CAD build for the part. Positions are in the model's coordinates, mm. A direction names the side the tool comes from. Round coordinates to 2 decimals unless told otherwise and drop trailing zeros. Loops run counter-clockwise (first coordinate to the right, second up) from the corner with the lowest first, then second, coordinate; pieces in that order, holes last.
from build123d import *

# Parameters (mm, degrees)
SKETCH1_R      = 53.975
SKETCH1_R_2    = 50.8
EXTRUDE1_DEPTH = 304.8
SKETCH2_W      = 76.2
SKETCH2_H      = 203.2
EXTRUDE2_DEPTH = 315.212732476
FILLET1_R      = 6.35


with BuildPart() as part:
    # Sketch1 → Extrude1 (new body)
    with BuildSketch(Plane.XY):
        with Locations(Location((0, 0, 0), (0, 0, 180))):
            Circle(SKETCH1_R)
        with Locations(Location((0, 0, 0), (0, 0, 180))):
            Circle(SKETCH1_R_2, mode=Mode.SUBTRACT)
    extrude(amount=EXTRUDE1_DEPTH)

    # Sketch2 → Extrude2 (cut, through all)
    with BuildSketch(Plane(origin=(0, 0, 0), x_dir=(1, 0, 0), z_dir=(0, 1, 0))):
        with Locations((0, -152.4)):
            Rectangle(SKETCH2_W, SKETCH2_H)
    extrude(amount=-EXTRUDE2_DEPTH, mode=Mode.SUBTRACT)

    # Fillet1
    # the kernel refuses this fillet: 6.35 mm, written as the material it adds along each edge
    with BuildSketch(Plane(origin=(-38.1, -17.726041651, 254), x_dir=(0, 0, -1), z_dir=(0, -1, 0))) as fillet1_piece_1_section:
        with BuildLine():
            CenterArc((FILLET1_R, FILLET1_R), FILLET1_R, 180, 90)
            Line((0, FILLET1_R), (0, 0))
            Line((0, 0), (FILLET1_R, 0))
        make_face()
    fillet1_piece_1 = extrude(amount=36.381021137, mode=Mode.PRIVATE)
    fillet1_piece_1 = fillet1_piece_1 & Plane(origin=(0, 0, 252.560306593), x_dir=(-1, 0, 0), z_dir=(0, 0, -1)) * Cylinder(53.975, 99, mode=Mode.PRIVATE)
    fillet1_piece_1 = fillet1_piece_1 - Plane(origin=(0, 0, 252.560306593), x_dir=(-1, 0, 0), z_dir=(0, 0, -1)) * Cylinder(50.8, 99, mode=Mode.PRIVATE)
    add(fillet1_piece_1)
    with BuildSketch(Plane(origin=(-38.1, -17.726041651, 50.8), x_dir=(1, 0, 0), z_dir=(0, -1, 0))) as fillet1_piece_2_section:
        with BuildLine():
            CenterArc((FILLET1_R, FILLET1_R), FILLET1_R, 180, 90)
            Line((0, FILLET1_R), (0, 0))
            Line((0, 0), (FILLET1_R, 0))
        make_face()
    fillet1_piece_2 = extrude(amount=36.381021137, mode=Mode.PRIVATE)
    fillet1_piece_2 = fillet1_piece_2 & Plane(origin=(0, 0, 52.23969466), x_dir=(-1, 0, 0), z_dir=(0, 0, -1)) * Cylinder(53.975, 99, mode=Mode.PRIVATE)
    fillet1_piece_2 = fillet1_piece_2 - Plane(origin=(0, 0, 52.23969466), x_dir=(-1, 0, 0), z_dir=(0, 0, -1)) * Cylinder(50.8, 99, mode=Mode.PRIVATE)
    add(fillet1_piece_2)
    with BuildSketch(Plane(origin=(38.1, -17.726041651, 50.8), x_dir=(-1, 0, 0), z_dir=(0, -1, 0))) as fillet1_piece_3_section:
        with BuildLine():
            CenterArc((FILLET1_R, -FILLET1_R), FILLET1_R, 90, 90)
            Line((0, -FILLET1_R), (0, 0))
            Line((0, 0), (FILLET1_R, 0))
        make_face()
    fillet1_piece_3 = extrude(amount=36.381021137, mode=Mode.PRIVATE)
    fillet1_piece_3 = fillet1_piece_3 & Plane(origin=(0, 0, 52.239693302), x_dir=(-1, 0, 0), z_dir=(0, 0, -1)) * Cylinder(53.975, 99, mode=Mode.PRIVATE)
    fillet1_piece_3 = fillet1_piece_3 - Plane(origin=(0, 0, 52.239693302), x_dir=(-1, 0, 0), z_dir=(0, 0, -1)) * Cylinder(50.8, 99, mode=Mode.PRIVATE)
    add(fillet1_piece_3)
    with BuildSketch(Plane(origin=(38.1, -17.726041651, 254), x_dir=(-1, 0, 0), z_dir=(0, -1, 0))) as fillet1_piece_4_section:
        with BuildLine():
            CenterArc((FILLET1_R, FILLET1_R), FILLET1_R, 180, 90)
            Line((0, FILLET1_R), (0, 0))
            Line((0, 0), (FILLET1_R, 0))
        make_face()
    fillet1_piece_4 = extrude(amount=36.381021137, mode=Mode.PRIVATE)
    fillet1_piece_4 = fillet1_piece_4 & Plane(origin=(0, 0, 252.560306698), x_dir=(-1, 0, 0), z_dir=(0, 0, -1)) * Cylinder(53.975, 99, mode=Mode.PRIVATE)
    fillet1_piece_4 = fillet1_piece_4 - Plane(origin=(0, 0, 252.560306698), x_dir=(-1, 0, 0), z_dir=(0, 0, -1)) * Cylinder(50.8, 99, mode=Mode.PRIVATE)
    add(fillet1_piece_4)


solid = part.part
Item 1: Cut at D-D (z = 175). List the corners of the cut face in (x, y) (3 decimals), plus the area to 3 significant figures.
Verdict:
outline: (-38.1, -38.232) - (-38.1, -33.601) arc R50.8 cw (long way) to (38.1, -33.601) - (38.1, -38.232) arc R53.975 ccw (long way) to start
area: 774 mm2
Item 2: Cut at C-C (x = 41). List the corners of the cut face in (y, z).
Verdict:
outline: (-35.1, 0) - (-29.99, 0) - (-29.99, 304.8) - (-35.1, 304.8) - close; (29.99, 0) - (35.1, 0) - (35.1, 304.8) - (29.99, 304.8) - close
Item 3: Cut at A-A (y = 0). List the corners of the cut face in (x, z) (3 decimals), plus the area to 3 significant figures.
Verdict:
outline: (-53.975, 0) - (-50.8, 0) - (-50.8, 304.8) - (-53.975, 304.8) - close; (50.8, 0) - (53.975, 0) - (53.975, 304.8) - (50.8, 304.8) - close
area: 1,940 mm2
Item 4: Cut at B-B (x = 0). List the corners of the cut face in (y, z) (3 decimals).
Verdict:
outline: (-53.975, 0) - (-50.8, 0) - (-50.8, 50.8) - (-53.975, 50.8) - close; (-53.975, 254) - (-50.8, 254) - (-50.8, 304.8) - (-53.975, 304.8) - close; (50.8, 0) - (53.975, 0) - (53.975, 304.8) - (50.8, 304.8) - close
Item 5: Wall check: L1, parallel to X at y = 0.5, z = 205; L2, parallel to X at y = -5.5, z = 186; L3, parallel to Y at x = 1, z = 276. Give the ranges that are in metal, low to high.
Verdict:
L1: x = -53.97 to -50.8, 50.8 to 53.97
L2: x = -53.69 to -50.5, 50.5 to 53.69
L3: y = -53.97 to -50.79, 50.79 to 53.97
Item 6: Mould opens along Z. For faces 3 (the flat face through (-40, 32, 0)), 4 (the flat face through (0, -52, 50.8)), 5 (the flat face through (-40, 32, 304.8)) say: released by +Z, released by -Z, zero draft, split by the parting line, or undercut.
Verdict:
face 3: released by -Z
face 4: undercut
face 5: released by +Z
Item 7: 3-axis set-ups, long thin cutter, end or side, ignore diameter. For faces 1 (the cylindrical face through (36.19, -38.55, 52.61)), 2 (the cylindrical face through (7.026, 53.516, 150.266)): which of +Z, -Z, +X, -X, +Y, -Y reach the whole face in a straight line?
Verdict:
face 1: -Y
face 2: +Z, -Z
Item 8: Flat gauge pins, fed straight in: P1, Ø4, axis at x = 22.5, z = 90.5, coming from the -Y side; P2, Ø5, axis at y = 26, z = 251.5, coming from the -X side; P3, Ø2.5, axis at y = -35.5, z = 170, coming from the -X side. Where does each tip first touch, or does it go through?
Verdict:
P1: stops at y = 44.5
P2: stops at x = -48.59
P3: stops at x = -41.72
